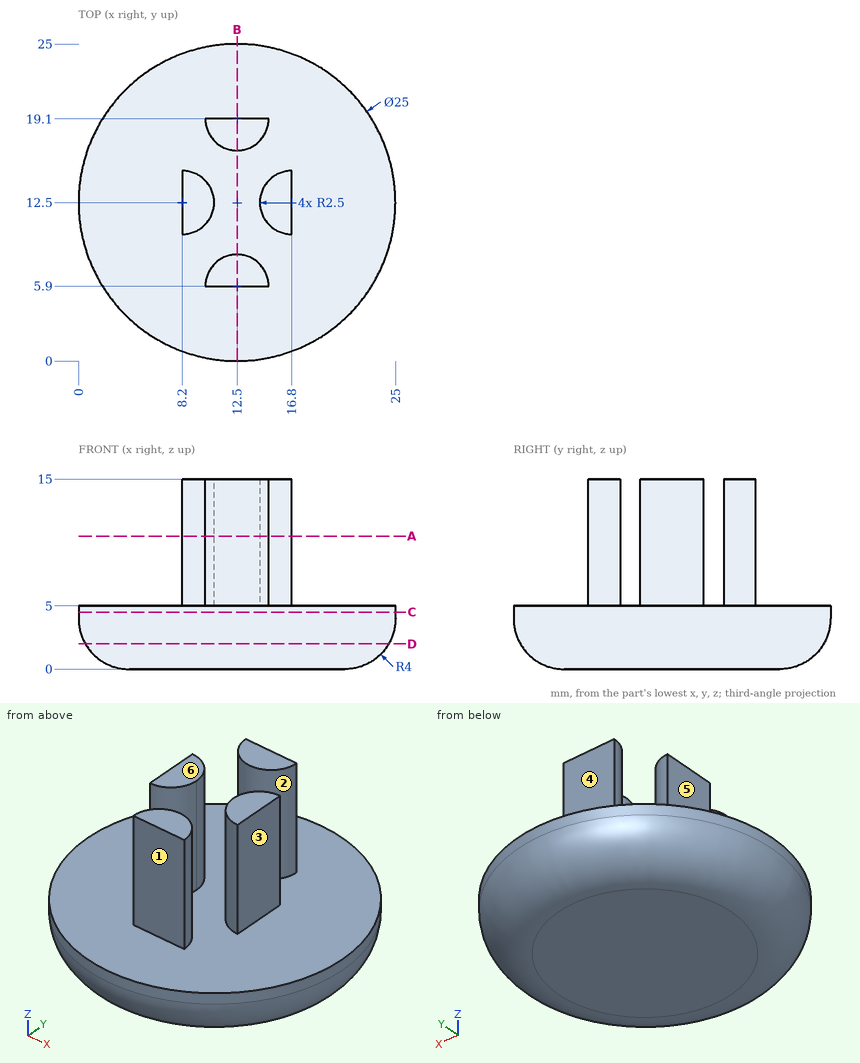
Source: three-view drawing plus pictorial views. Frame: mm from the lowest corner of the part. A direction names the side the tool comes from. Round coordinates to 2 decimals unless told otherwise and drop trailing zeros. Order: outer loops, then holes, each group sorted by start corner. A loop starts at its lowest first (then second) coordinate and runs counter-clockwise, first axis right, second up. Notation, with made-up numbers: (66, 42.25) - (95, 42.25) arc R22 ccw to (95, 59.25) - close; hole circle Ø11 at (64, 74). An arc over 180 degrees is marked (long way). Use a Markdown table: item, result.
1. Access query for the marked faces 4, 5 and 6. Directions: +Z, -Z, +X, -X, +Y, -Y. A direction counts if a zero-diameter tool reaches every point of the face in a straight line with its end or side. Return the directions, or none.
Evaluation:
| item | result |
|---|---|
| face 4 | +Z, +X, -X, +Y |
| face 5 | +Z, -X, +Y, -Y |
| face 6 | +Z, +X, -X, +Y, -Y |
2. Section C-C on z = 4.5. Return the cut outline in (x, y).
Evaluation:
| item | result |
|---|---|
| outline | circle Ø25 at (12.5, 12.5) |
3. Mould query, pull axis Y, two halves, no side actions, for the marked faces 1, 2 and 3. Classes: +Y half, -Y half, draft (parallel to the pull), parting line (faces both ways), or undercut.
Evaluation:
| item | result |
|---|---|
| face 1 | -Y half |
| face 2 | undercut |
| face 3 | draft |
4. Material intervals for probe 1 along Z at (x, y) = (18.75, 10.25); probe 2 along Y at (x, z) = (10.25, 11.5); probe 3 along X at (y, z) = (22.25, 4.25), sorted ascending.
Evaluation:
| item | result |
|---|---|
| probe 1 | 0 to 5 |
| probe 2 | 5.9 to 6.99, 11.07 to 13.93, 18.01 to 19.1 |
| probe 3 | 4.68 to 20.32 |
5. Section D-D on z = 2. Return the cut outline in (x, y), then the cut area to 3 significant figures.
Evaluation:
| item | result |
|---|---|
| outline | circle Ø23.93 at (12.5, 12.5) |
| area | 450 mm^2 |
6. Section A-A on z = 10.5. Return the cut outline in (x, y).
Evaluation:
| item | result |
|---|---|
| outline | (8.2, 10) arc R2.5 ccw to (8.2, 15) - close; (10, 5.9) - (15, 5.9) arc R2.5 ccw to start; (10, 19.1) arc R2.5 ccw to (15, 19.1) - close; (16.8, 10) - (16.8, 15) arc R2.5 ccw to start |
7. Section B-B on x = 12.5. Return the cut outline in (y, z).
Evaluation:
| item | result |
|---|---|
| outline | (0, 4) arc R4 ccw to (4, 0) - (21, 0) arc R4 ccw to (25, 4) - (25, 5) - (19.1, 5) - (19.1, 15) - (16.6, 15) - (16.6, 5) - (8.4, 5) - (8.4, 15) - (5.9, 15) - (5.9, 5) - (0, 5) - close |
8. First-contact query: pin 1 (4 mm diameter, centred on x = 18.5, y = 4, fed in from -Z); pin 2 (4 mm diameter, centred on x = 5.5, y = 13, fed in from +Z); pin 3 (2.5 mm diameter, centred on x = 13, z = 9.5, fed in from +Y); pin 4 (4 mm diameter, centred on y = 13, z = 7.5, fed in from -X). Flat tips, straight axial feed; report the tip coordinate or a pass-through.
Evaluation:
| item | result |
|---|---|
| pin 1 | z = 0 |
| pin 2 | z = 5 |
| pin 3 | y = 19.1 |
| pin 4 | x = 8.2 |
